Check sheet for the modelled part. Datum: model origin and axes. Units: mm. A direction names the side the tool comes from. Round coordinates to 2 decimals unless told otherwise and drop trailing zeros. Order: outer loops, then holes, each group sorted by start corner. A loop starts at its lowest first (then second) coordinate and runs counter-clockwise, first axis right, second up.
Autodesk Fusion 360 part; units mm, degrees
sketch "Sketch1" plane through (0, 0, 0) normal (0, 1, 0) x (1, 0, 0)
  circle A0 centre (0, 0) radius 25.4
  dimension "d1" = 50.8
extrude "Extrude1" add sketch "Sketch1" along normal blind 12.7
sketch "Sketch2" plane through (0, 12.7, 0) normal (0, 1, 0) x (-1, 0, 0)
  circle A0 centre (0, 0) radius 25.4
  circle A1 centre (0, -25.4) radius 6.35
  dimension "d4" = 12.7
extrude "Extrude2" cut sketch "Sketch2" against normal blind 6.35 contours A0 A1 | A0 A1 picked at (-1.9477, -23.4128) picked at (2.1308, -27.1585)
sketch "Sketch3" plane through (0, 12.7, 0) normal (0, 1, 0) x (-1, 0, 0)
  arc A0 (6.3002, -24.6062) -> (-6.3002, -24.6062) centre (0, -25.4) ccw
  arc A1 (6.3002, -24.6063) -> (-6.3002, -24.6062) centre (0, 0) ccw
  circle A2 centre (0, -10.795) radius 4.7625
  circle A3 centre (0, -10.795) radius 2.5527
  dimension "d7" = 9.525
  dimension "d8" = 10.795
  dimension "d9" = 5.1054
sketch "Sketch4" plane through (0, 0, 0) normal (1, 0, 0) x (0, 0, -1)
  line L0 (25.4, 0) -> (25.4, 6.35)
  line L1 (-25.4, 12.7) -> (-25.4, 0)
  line L2 (19.05, 6.35) -> (24.6062, 6.35)
  line L3 (25.4, 6.35) -> (22.225, 6.35)
  line L4 (22.225, 7.9375) -> (25.4, 7.9375)
  line L5 (25.4, 7.9375) -> (25.4, 6.35)
  line L6 (22.225, 7.9375) -> (22.225, 6.35)
  dimension "d12" = 3.175
  dimension "d13" = 1.5875
revolve "Revolve1" cut sketch "Sketch4" angle 360 about axis through (0, 1.75, 0) along (0, 1, 0)
1) Sectioned sample at D-D on z = -12.5. Record the cut outline in (x, y).
2) Gauge pin test, flat ends, axial feed: pin 1 (1 mm diameter, centred on y = 7, z = 12, fed in from -X); pin 2 (3 mm diameter, centred on x = -16.5, y = 8.5, fed in from -Z); pin 3 (2 mm diameter, centred on x = 3.5, y = 8, fed in from +Z). Record the tip position at first contact, or that the pin passes through.
3) Scan lines: line 1 (Y direction, x = -12, z = -20); line 2 (Z direction, x = 0, y = 2.25); line 3 (X direction, y = 10, z = 1). Record each from-to range of solid material in increasing order.
4) Draft check along X on faces 3 (the face through (0, 0, 0)), 4 (the face through (-5.506, 3.131, -24.796)), 5 (the face through (-0.13, 9.57, -19.05)). Enter one of: pulls with the +X half, pulls with the -X half, needs draft (parallel to the pull), parting line crosses it, or undercut.
5) Sectioned sample at C-C on y = 4.25. Record the cut outline in (x, z).
6) Set-up check for faces 1 (the face through (0, 7.938, 23)), 2 (the face through (1.03, 10.29, 25.38)): record each of +Z, -Z, +X, -X, +Y, -Y from which the full face is reachable in a straight line by a thin tool's end or side.
Values found:
1. outline: (-22.11, 0) - (22.11, 0) - (22.11, 6.35) - (18.38, 6.35) - (18.38, 7.94) - (22.11, 7.94) - (22.11, 12.7) - (-22.11, 12.7) - (-22.11, 7.94) - (-18.38, 7.94) - (-18.38, 6.35) - (-22.11, 6.35) - close
2. pin 1: stops at x = -19.02
2. pin 2: stops at z = -20.5
2. pin 3: stops at z = 25.28
3. line 1: y = 0 to 6.35, 7.94 to 12.7
3. line 2: z = -25.4 to 25.4
3. line 3: x = -25.38 to 25.38
4. face 3: needs draft
4. face 4: parting line crosses it
4. face 5: undercut
5. outline: circle Ø50.8 at (0, 0)
6. face 1: none
6. face 2: +Y, -Y
